The model under review builds one solid part; all positions refer to its coordinate system, in mm. Round coordinates to 2 decimals unless told otherwise and drop trailing zeros. Loops run counter-clockwise (first coordinate to the right, second up) from the corner with the lowest first, then second, coordinate; pieces in that order, holes last. Notation, with made-up numbers: (66, 36.5) -> (81, 36.5) arc R31 cw to (81, 63.5) -> close; hole circle Ø6 at (16, -26.75). An arc over 180 degrees is marked (long way). Use a Markdown table: item, result. Add a question column.
1) Consider section C-C on z = 1. State how many separate pieces and enclosed holes the cut face has, plus the area to 3 significant figures.
2) Insertion check: pin 1 (0.9 mm diameter, centred on x = 55, z = 1, fed in from +Y); pin 2 (0.9 mm diameter, centred on x = 19.5, z = 1, fed in from +Y); pin 3 (5 mm diameter, centred on x = 56.88, y = 255.91, fed in from +Z); pin 4 (10 mm diameter, centred on x = 53, y = 246, fed in from +Z). Each pin has a flat end and moves straight along its axis. Give the tip position at first contact, or say it passes through.
3) Consider section B-B on y = 246. Give the boundary of the cut face in (x, z), plus the area to 3 significant figures.
4) Wall thickness on probe 1 along Y at (x, z) = (32, 1.75); probe 2 along Y at (x, z) = (56.5, 1.7); probe 3 along X at (y, z) = (241.5, 2.55): over which ranges is each line inside the solid? List them lowest first.
5) Consider section A-A on x = 34. Give the boundary of the cut face in (y, z), plus the area to 3 significant figures.
from build123d import *

# Parameters (mm, degrees)
MODEL_R                 = 1.5
SALIENTE_EXTRUIR1_DEPTH = 3


with BuildPart() as part:
    # Model → Saliente-Extruir1 (new body)
    with BuildSketch(Plane.XY):
        with BuildLine():
            ThreePointArc((59.248437734, 226.067919021), (60.634120255, 227.670602527), (61.132865862, 229.729719641))
            Line((61.132865862, 229.729719641), (61.132865862, 282.097548174))
            ThreePointArc((61.132865862, 282.097548174), (60.634120255, 284.156665288), (59.248437734, 285.759348794))
            Line((59.248437734, 285.759348794), (51.806344994, 291.075129323))
            ThreePointArc((51.806344994, 291.075129323), (50.564071562, 291.698658491), (49.190773122, 291.913328703))
            Line((49.190773122, 291.913328703), (25.074958603, 291.913328703))
            ThreePointArc((25.074958603, 291.913328703), (23.701660163, 291.698658491), (22.459386731, 291.075129323))
            Line((22.459386731, 291.075129323), (15.017293991, 285.759348794))
            ThreePointArc((15.017293991, 285.759348794), (13.63161147, 284.156665288), (13.132865862, 282.097548174))
            Line((13.132865862, 282.097548174), (13.132865862, 229.729719641))
            ThreePointArc((13.132865862, 229.729719641), (13.63161147, 227.670602527), (15.017293991, 226.067919021))
            Line((15.017293991, 226.067919021), (22.459386731, 220.752138492))
            ThreePointArc((22.459386731, 220.752138492), (23.701660163, 220.128609324), (25.074958603, 219.913939113))
            Line((25.074958603, 219.913939113), (49.190773122, 219.913939113))
            ThreePointArc((49.190773122, 219.913939113), (50.564071562, 220.128609324), (51.806344994, 220.752138492))
            Line((51.806344994, 220.752138492), (59.248437734, 226.067919021))
        make_face()
        with Locations((28.132865862, 224.413939113)):
            Circle(MODEL_R, mode=Mode.SUBTRACT)
        with BuildLine():
            ThreePointArc((20.454104838, 256.369594574), (23.38312543, 255.913735735), (20.454166764, 255.457479185))
            ThreePointArc((20.454166764, 255.457479185), (14.28786587, 255.913118236), (20.454104838, 256.369594574))
        make_face(mode=Mode.SUBTRACT)
        with Locations((37.132865862, 224.413939113)):
            Circle(MODEL_R, mode=Mode.SUBTRACT)
        with Locations((46.132865862, 224.413939113)):
            Circle(MODEL_R, mode=Mode.SUBTRACT)
        with BuildLine():
            ThreePointArc((53.811907003, 255.45692477), (50.883125437, 255.913735745), (53.81196901, 256.370148994))
            ThreePointArc((53.81196901, 256.370148994), (59.978125426, 255.913118206), (53.811907003, 255.45692477))
        make_face(mode=Mode.SUBTRACT)
        with Locations((28.132865862, 287.413939112)):
            Circle(MODEL_R, mode=Mode.SUBTRACT)
        with BuildLine():
            Line((16.132865862, 263.413328703), (16.132865862, 281.413328703))
            ThreePointArc((16.132865862, 281.413328703), (16.572205691, 282.473988875), (17.632865862, 282.913328703))
            Line((17.632865862, 282.913328703), (56.632865862, 282.913328703))
            ThreePointArc((56.632865862, 282.913328703), (57.693526034, 282.473988875), (58.132865862, 281.413328703))
            Line((58.132865862, 281.413328703), (58.132865862, 263.413328703))
            ThreePointArc((58.132865862, 263.413328703), (57.693526034, 262.352668531), (56.632865862, 261.913328703))
            Line((56.632865862, 261.913328703), (53.293383336, 261.913328703))
            Line((53.293383336, 261.913328703), (53.172348389, 261.913328703))
            ThreePointArc((53.172348389, 261.913328703), (47.235274136, 256.083614768), (52.832637551, 249.926997348))
            Line((52.832637551, 249.926997348), (56.632865862, 249.926997348))
            ThreePointArc((56.632865862, 249.926997348), (57.693526034, 249.48765752), (58.132865862, 248.426997348))
            Line((58.132865862, 248.426997348), (58.132865862, 230.413939113))
            ThreePointArc((58.132865862, 230.413939113), (57.693526034, 229.353278941), (56.632865862, 228.913939113))
            Line((56.632865862, 228.913939113), (17.632865862, 228.913939113))
            ThreePointArc((17.632865862, 228.913939113), (16.572205691, 229.353278941), (16.132865862, 230.413939113))
            Line((16.132865862, 230.413939113), (16.132865862, 248.426997348))
            ThreePointArc((16.132865862, 248.426997348), (16.572205691, 249.48765752), (17.632865862, 249.926997348))
            Line((17.632865862, 249.926997348), (21.433094174, 249.926997348))
            ThreePointArc((21.433094174, 249.926997348), (27.030457589, 256.083614768), (21.093383336, 261.913328703))
            Line((21.093383336, 261.913328703), (20.972348389, 261.913328703))
            Line((20.972348389, 261.913328703), (17.632865862, 261.913328703))
            ThreePointArc((17.632865862, 261.913328703), (16.572205691, 262.352668531), (16.132865862, 263.413328703))
        make_face(mode=Mode.SUBTRACT)
        with Locations((37.132865862, 287.413939112)):
            Circle(MODEL_R, mode=Mode.SUBTRACT)
        with Locations((46.132865862, 287.413939112)):
            Circle(MODEL_R, mode=Mode.SUBTRACT)
    extrude(amount=SALIENTE_EXTRUIR1_DEPTH)


solid = part.part
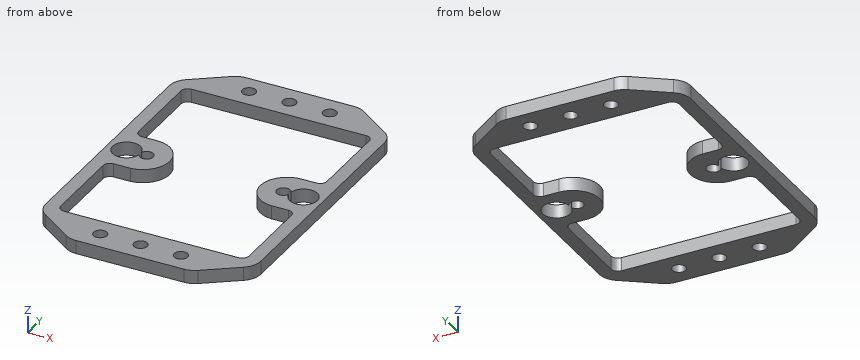
Result set:
| question | item | result |
|---|---|---|
| 1 | separate pieces | 1 |
| 1 | enclosed holes | 9 |
| 1 | area | 1,140 mm2 |
| 2 | pin 1 | y = 289.12 |
| 2 | pin 2 | y = 289.28 |
| 2 | pin 3 | through |
| 2 | pin 4 | z = 3 |
| 3 | outline | (13.13, 0) -> (16.13, 0) -> (16.13, 3) -> (13.13, 3) -> close; (58.13, 0) -> (61.13, 0) -> (61.13, 3) -> (58.13, 3) -> close |
| 3 | area | 18.0 mm2 |
| 4 | probe 1 | 219.91 to 228.91, 282.91 to 291.91 |
| 4 | probe 2 | 224.1 to 228.91, 249.93 to 252.84, 258.99 to 261.91, 282.91 to 287.72 |
| 4 | probe 3 | 13.13 to 16.13, 58.13 to 61.13 |
| 5 | outline | (219.91, 0) -> (228.91, 0) -> (228.91, 3) -> (219.91, 3) -> close; (282.91, 0) -> (291.91, 0) -> (291.91, 3) -> (282.91, 3) -> close |
| 5 | area | 54.0 mm2 |
